Model file for the job. Use its own axes, mm. Coordinates: 2 decimals unless noted, no trailing zeros. Order: outer loops, then holes, each group sorted by start corner. A loop starts at its lowest first (then second) coordinate and runs counter-clockwise, first axis right, second up. Notation, with made-up numbers: M 48.25,75.5 L 77.25,75.5 A37 cw 77.25,114.5 Z; hole C -40,78.25 d5. An arc over 180 degrees is marked long. Return JSON: item names as keys, results as strings.
```python
from build123d import *

# Parameters (mm, degrees)
BOSS_EXTRUDE1_DEPTH = 1.11
SKETCH3_R           = 2.6
SKETCH3_R_2         = 1.6
CUT_EXTRUDE5_DEPTH  = 12.11
SKETCH4_R           = 3.1
CUT_EXTRUDE6_DEPTH  = 2.11
SKETCH5_R           = 3.1
CUT_EXTRUDE7_DEPTH  = 2.11
SKETCH6_W           = 6.2
SKETCH6_H           = 6
SKETCH6_W_2         = 10.7
CUT_EXTRUDE8_DEPTH  = 2.11
FILLET1_R           = 1


with BuildPart() as part:
    # Sketch1 → Boss-Extrude1 (new body)
    with BuildSketch(Plane(origin=(0, 0, 0), x_dir=(1, 0, 0), z_dir=(0, 1, 0))):
        with BuildLine():
            Line((-66.5, -17), (66.5, -17))
            ThreePointArc((66.5, -17), (68.267766953, -16.267766953), (69, -14.5))
            Line((69, -14.5), (69, 14.5))
            ThreePointArc((69, 14.5), (68.267766953, 16.267766953), (66.5, 17))
            Line((66.5, 17), (-66.5, 17))
            ThreePointArc((-66.5, 17), (-68.267766953, 16.267766953), (-69, 14.5))
            Line((-69, 14.5), (-69, -14.5))
            ThreePointArc((-69, -14.5), (-68.267766953, -16.267766953), (-66.5, -17))
        make_face()
    extrude(amount=BOSS_EXTRUDE1_DEPTH)

    # Sketch3 → Cut-Extrude5 (cut, through all)
    with BuildSketch(Plane(origin=(0, -10, 0), x_dir=(1, 0, 0), z_dir=(0, 1, 0))):
        with Locations((-52, 0)):
            Circle(SKETCH3_R)
        with Locations((52, 0)):
            Circle(SKETCH3_R)
        with Locations((-52, 12)):
            Circle(SKETCH3_R_2)
        with Locations((-52, -12)):
            Circle(SKETCH3_R_2)
        with Locations((52, -12)):
            Circle(SKETCH3_R_2)
        with Locations((52, 12)):
            Circle(SKETCH3_R_2)
        with Locations((-64, 0)):
            Circle(SKETCH3_R_2)
        with Locations((64, 0)):
            Circle(SKETCH3_R_2)
    extrude(amount=CUT_EXTRUDE5_DEPTH, mode=Mode.SUBTRACT)

    # Sketch4 → Cut-Extrude6 (cut, through all)
    with BuildSketch(Plane.XZ):
        with Locations((0, 11.655)):
            Circle(SKETCH4_R)
        with Locations((-12, 11.655)):
            Circle(SKETCH4_R)
    extrude(amount=-CUT_EXTRUDE6_DEPTH, mode=Mode.SUBTRACT)

    # Sketch5 → Cut-Extrude7 (cut, through all)
    with BuildSketch(Plane.XZ):
        with Locations((-16.5, 11.655)):
            Circle(SKETCH5_R)
        with Locations((-28.5, 11.655)):
            Circle(SKETCH5_R)
        with Locations((28.5, 11.655)):
            Circle(SKETCH5_R)
        with Locations((16.5, 11.655)):
            Circle(SKETCH5_R)
    extrude(amount=-CUT_EXTRUDE7_DEPTH, mode=Mode.SUBTRACT)

    # Sketch6 → Cut-Extrude8 (cut, through all)
    with BuildSketch(Plane(origin=(0, 1.11, 0), x_dir=(1, 0, 0), z_dir=(0, 1, 0))):
        with Locations((-28.5, -14.655)):
            Rectangle(SKETCH6_W, SKETCH6_H)
        with Locations((-14.25, -14.655)):
            Rectangle(SKETCH6_W_2, SKETCH6_H)
        with Locations((0, -14.655)):
            Rectangle(SKETCH6_W, SKETCH6_H)
        with Locations((28.5, -14.655)):
            Rectangle(SKETCH6_W, SKETCH6_H)
        with Locations((16.5, -14.655)):
            Rectangle(SKETCH6_W, SKETCH6_H)
    extrude(amount=-CUT_EXTRUDE8_DEPTH, mode=Mode.SUBTRACT)

    # Fillet1
    fillet1_edges = [part.edges().sort_by_distance(p)[0] for p in [
        (-31.6, 0.555, 17),
        (-25.4, 0.555, 17),
        (-8.9, 0.555, 17),
        (-19.6, 0.555, 17),
        (-3.1, 0.555, 17),
        (3.1, 0.555, 17),
        (25.4, 0.555, 17),
        (31.6, 0.555, 17),
        (13.4, 0.555, 17),
        (19.6, 0.555, 17),
    ]]
    fillet(fillet1_edges, radius=FILLET1_R)


solid = part.part
```
Item 1: Pull direction Y, two halves, no side cores. Call faces 1 (the cylindrical face through (-10.9, 0.547, 8.757)), 2 (the flat face through (-1, 0, 0)): +Y half, -Y half, draft (parallel to the pull), parting line (faces both ways), or undercut.
Check result:
{"face 1": "draft", "face 2": "-Y half"}
Item 2: Drop flat-ended pins along their axis: pin 1 Ø1.9 at (x, z) = (-64, 0) entering from -Y; pin 2 Ø8.5 at (x, z) = (-52, 0) entering from -Y. Give the stop position or say it passes through.
Check result:
{"pin 1": "passes through", "pin 2": "stops at y = 0"}
Item 3: Saw through at A-A (x = -64). Write the cut outline in (y, z), and give its area (3 significant figures).
Check result:
{"outline": "M 0,-17 L 1.11,-17 L 1.11,-1.6 L 0,-1.6 Z; M 0,1.6 L 1.11,1.6 L 1.11,17 L 0,17 Z", "area": "34.2 mm2"}
Item 4: Saw through at C-C (x = 52). Write the cut outline in (y, z), and give its area (3 significant figures).
Check result:
{"outline": "M 0,-17 L 1.11,-17 L 1.11,-13.6 L 0,-13.6 Z; M 0,-10.4 L 1.11,-10.4 L 1.11,-2.6 L 0,-2.6 Z; M 0,2.6 L 1.11,2.6 L 1.11,10.4 L 0,10.4 Z; M 0,13.6 L 1.11,13.6 L 1.11,17 L 0,17 Z", "area": "24.9 mm2"}
Item 5: Saw through at D-D (z = 0). Write the cut outline in (x, y), and give its area (3 significant figures).
Check result:
{"outline": "M -69,0 L -65.6,0 L -65.6,1.11 L -69,1.11 Z; M -62.4,0 L -54.6,0 L -54.6,1.11 L -62.4,1.11 Z; M -49.4,0 L 49.4,0 L 49.4,1.11 L -49.4,1.11 Z; M 54.6,0 L 62.4,0 L 62.4,1.11 L 54.6,1.11 Z; M 65.6,0 L 69,0 L 69,1.11 L 65.6,1.11 Z", "area": "135 mm2"}
Item 6: Saw through at B-B (z = -12). Write the cut outline in (x, y), and give its area (3 significant figures).
Check result:
{"outline": "M -69,0 L -53.6,0 L -53.6,1.11 L -69,1.11 Z; M -50.4,0 L 50.4,0 L 50.4,1.11 L -50.4,1.11 Z; M 53.6,0 L 69,0 L 69,1.11 L 53.6,1.11 Z", "area": "146 mm2"}
Item 7: Wall check: line 1 (Z direction, x = -52, y = 0.6); line 2 (Z direction, x = -64, y = 0.7); line 3 (X direction, y = 0.8, z = 2). Give the ranges that are in metal, low to high.
Check result:
{"line 1": "z = -17 to -13.6, -10.4 to -2.6, 2.6 to 10.4, 13.6 to 17", "line 2": "z = -17 to -1.6, 1.6 to 17", "line 3": "x = -69 to -53.66, -50.34 to 50.34, 53.66 to 69"}
